The listing builds one solid part. Answer for the finished solid, in the listing's coordinates (mm). Face numbers are marked on the shaded views. A direction names the side the tool comes from. Round coordinates to 2 decimals unless told otherwise and drop trailing zeros. Loops run counter-clockwise (first coordinate to the right, second up) from the corner with the lowest first, then second, coordinate; pieces in that order, holes last. Notation, with made-up numbers: (13, 19.5) -> (70, 19.5) arc R23 ccw to (70, 52.5) -> close; hole circle Ø10 at (-11.75, 29.5). An arc over 180 degrees is marked (long way). Use a Markdown table: item, result. Add a question column.
Q1. Section C-C on z = -112.5 is taken. Give the vertices of the cut face in (x, y).
Q2. Section A-A on z = 0 is taken. Give the vertices of the cut face in (x, y).
Q3. Given pin 1 Ø3 at (y, z) = (4, -59.5) entering from -X; pin 2 Ø3 at (x, y) = (12.5, 10) entering from -Z; pin 3 Ø1.5 at (x, y) = (23.5, 10.5) entering from +Z; pin 4 Ø8 at (x, z) = (18.5, -53.5) entering from -Y, each flat-ended and moving along its own axis, determine where each tip first touches the part or whether it passes through.
Q4. Section B-B on x = 0 is taken. Give the vertices of the cut face in (y, z), then the cut area to 3 significant figures.
Q5. Consider line 1 (X direction, y = 9.25, z = 0); line 2 (X direction, y = 5, z = -112.5); line 3 (Z direction, x = 1, y = 3.75). Determine where each line is inside the solid, lowest interval first.
Q6. Section D-D on x = 65 is taken. Give the vertices of the cut face in (y, z).
Q7. For a pull along Z with two mould halves and no side action, classify the marked faces 4, 5, 6 and 7 as released by +Z, released by -Z, zero draft, split by the parting line, or undercut.
Q8. Which of the six approach directions +Z, -Z, +X, -X, +Y, -Y give full straight-line access (tool end or side, diameter ignored) to the marked faces 1, 2 and 3?
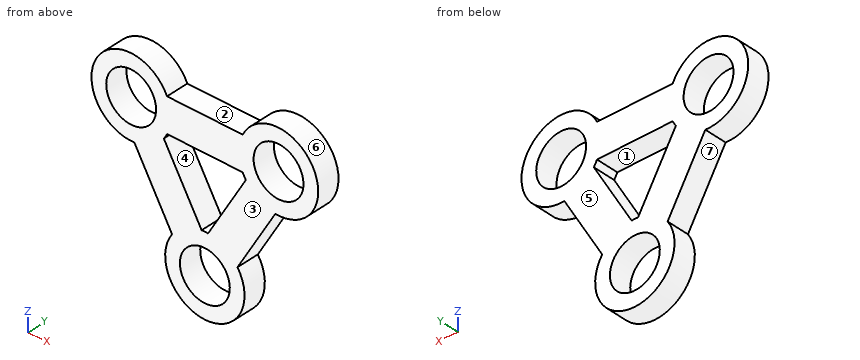
from build123d import *

# Parameters (mm, degrees)
SKETCH1_R           = 22
BOSS_EXTRUDE1_DEPTH = 20


with BuildPart() as part:
    # Sketch1 → Boss-Extrude1 (new body)
    with BuildSketch(Plane(origin=(0, 0, 0), x_dir=(1, 0, 0), z_dir=(0, 1, 0))):
        with BuildLine():
            Line((98.377223398, -15), (31.622776602, -15))
            ThreePointArc((31.622776602, -15), (-30.313693749, -17.495141363), (2.832190618, 34.885221747))
            Line((2.832190618, 34.885221747), (36.097300033, 92.760852739))
            ThreePointArc((36.097300033, 92.760852739), (65.083539163, 147.499900303), (93.808142815, 92.62310619))
            Line((93.808142815, 92.62310619), (127.167809382, 34.885221747))
            ThreePointArc((127.167809382, 34.885221747), (160.313693749, -17.495141363), (98.377223398, -15))
        make_face()
        with Locations(Location((0, 0, 0), (0, 0, 270))):
            Circle(SKETCH1_R, mode=Mode.SUBTRACT)
        with Locations(Location((65, 112.5, 0), (0, 0, 270))):
            Circle(SKETCH1_R, mode=Mode.SUBTRACT)
        with Locations(Location((130, 0, 0), (0, 0, 270))):
            Circle(SKETCH1_R, mode=Mode.SUBTRACT)
        with BuildLine():
            Line((98.377223398, 15), (31.622776602, 15))
            ThreePointArc((31.622776602, 15), (30.313693749, 17.495141363), (28.808142815, 19.87689381))
            Line((28.808142815, 19.87689381), (62.167809382, 77.614778253))
            ThreePointArc((62.167809382, 77.614778253), (65, 77.5), (67.832190618, 77.614778253))
            Line((67.832190618, 77.614778253), (101.191857185, 19.87689381))
            ThreePointArc((101.191857185, 19.87689381), (99.686306251, 17.495141363), (98.377223398, 15))
        make_face(mode=Mode.SUBTRACT)
    extrude(amount=BOSS_EXTRUDE1_DEPTH)


solid = part.part
Checked values:
| question | item | result |
|---|---|---|
| 1 | outline | (30, 0) -> (43, 0) -> (43, 20) -> (30, 20) -> close; (87, 0) -> (100, 0) -> (100, 20) -> (87, 20) -> close |
| 2 | outline | (-35, 0) -> (-22, 0) -> (-22, 20) -> (-35, 20) -> close; (22, 0) -> (108, 0) -> (108, 20) -> (22, 20) -> close; (152, 0) -> (165, 0) -> (165, 20) -> (152, 20) -> close |
| 3 | pin 1 | stops at x = 16.12 |
| 3 | pin 2 | stops at z = -54.32 |
| 3 | pin 3 | stops at z = 26.6 |
| 3 | pin 4 | stops at y = 0 |
| 4 | outline | (0, -35) -> (20, -35) -> (20, -22) -> (0, -22) -> close; (0, 22) -> (20, 22) -> (20, 35) -> (0, 35) -> close |
| 4 | area | 520 mm2 |
| 5 | line 1 | x = -35 to -22, 22 to 108, 152 to 165 |
| 5 | line 2 | x = 30 to 43, 87 to 100 |
| 5 | line 3 | z = -34.99 to -21.98, 21.98 to 34.99 |
| 6 | outline | (0, -147.5) -> (20, -147.5) -> (20, -134.5) -> (0, -134.5) -> close; (0, -90.5) -> (20, -90.5) -> (20, -77.5) -> (0, -77.5) -> close; (0, -15) -> (20, -15) -> (20, 15) -> (0, 15) -> close |
| 7 | face 4 | undercut |
| 7 | face 5 | zero draft |
| 7 | face 6 | split by the parting line |
| 7 | face 7 | undercut |
| 8 | face 1 | +Y, -Y |
| 8 | face 2 | +Z, +Y, -Y |
| 8 | face 3 | +Z, -Z, +X, -X, -Y |
